```python
from build123d import *

# Parameters (mm, degrees)
SKETCH_1_R          = 4
EXTRUDE_1_DEPTH     = 6.6
SKETCH_2_R          = 4.55
EXTRUDE_2_DEPTH     = 0.2
SKETCH_5_W          = 0.8
SKETCH_5_H          = 0.992889455
EXTRUDE_4_DEPTH     = 0.2
SKETCH_4_R          = 2.4
CUT_EXTRUDE_1_DEPTH = 0.3
FILLET_1_R          = 0.5
SKETCH_3_R          = 0.125
EXTRUDE_3_DEPTH     = 8


with BuildPart() as part:
    # 草图1 → 凸台-拉伸1 (new body)
    with BuildSketch(Plane(origin=(0, 0, 0), x_dir=(1, 0, 0), z_dir=(0, 1, 0))):
        with Locations(Location((0, 0, 0), (0, 0, 270))):
            Circle(SKETCH_1_R)
    extrude(amount=EXTRUDE_1_DEPTH)

    # 草图2 → 凸台-拉伸2 (add)
    with BuildSketch(Plane.XZ):
        with Locations(Location((0, 0, 0), (0, 0, 270))):
            Circle(SKETCH_2_R)
    extrude(amount=EXTRUDE_2_DEPTH)

    # 草图5 → 凸台-拉伸4 (add)
    with BuildSketch(Plane.XZ.offset(0.2)):
        with Locations((0, 4.725827174)):
            Rectangle(SKETCH_5_W, SKETCH_5_H)
    extrude(amount=-EXTRUDE_4_DEPTH)

    # 草图4 → 切除-拉伸1 (cut)
    with BuildSketch(Plane(origin=(0, 6.6, 0), x_dir=(1, 0, 0), z_dir=(0, 1, 0))):
        with Locations(Location((0, 0, 0), (0, 0, 270))):
            Circle(SKETCH_4_R)
    extrude(amount=-CUT_EXTRUDE_1_DEPTH, mode=Mode.SUBTRACT)

    # 圆角1
    fillet_1_edges = [part.edges().sort_by_distance(p)[0] for p in [
        (0, 6.6, -4),
    ]]
    fillet(fillet_1_edges, radius=FILLET_1_R)

    # 草图3 → 凸台-拉伸3 (add)
    with BuildSketch(Plane.XZ.offset(0.2)):
        with Locations(Location((-1.55, 1.55, 0), (0, 0, 270))):
            Circle(SKETCH_3_R)
        with Locations(Location((1.55, 1.55, 0), (0, 0, 90))):
            Circle(SKETCH_3_R)
        with Locations(Location((1.55, -1.55, 0), (0, 0, 270))):
            Circle(SKETCH_3_R)
        with Locations(Location((-1.55, -1.55, 0), (0, 0, 90))):
            Circle(SKETCH_3_R)
    extrude(amount=EXTRUDE_3_DEPTH)


solid = part.part
```
Model file for the job. Use its own axes, mm. Coordinates: 2 decimals unless noted, no trailing zeros. Write each loop counter-clockwise with the first axis right and the second up, starting at its lowest first coordinate (ties: lowest second). Pieces come first, ordered by that corner, then holes. Notation, with made-up numbers: (55, 42.5) - (91, 42.5) arc R19 cw to (91, 66.5) - close; hole circle Ø8 at (-20.5, 83). An arc over 180 degrees is marked (long way). Use a Markdown table: item, result. Add a question column.
Item 1: Drop flat-ended pins along their axis: pin 1 (1.5 mm diameter, centred on x = 2.5, y = 2, fed in from -Z); pin 2 (3 mm diameter, centred on x = -3, z = 4, fed in from -Y); pin 3 (5 mm diameter, centred on x = -1.5, y = -2.5, fed in from +Z). Give the stop position or say it passes through.
Item 2: Band-saw the part on B-B, the plane y = -0.75. Write the cut outline in (x, z) (3 decimals), and give its area (3 significant figures).
Item 3: Two-plate mould, pull along X, no slides. Class faces 1 (the face through (2.04, 0, 3.62)), 2 (the face through (-3.905, 3.007, -0.867)), 3 (the face through (1.62, 6.45, -1.77)): pulls with the +X half, pulls with the -X half, needs draft (parallel to the pull), parting line crosses it, or undercut.
Item 4: Drill centre lines: line 1 along Y through (x, z) = (2.75, 0.75); line 2 along Y through (x, z) = (1.25, 1.5); line 3 along X through (y, z) = (6.4, 0). Where is each one in solid material? Low to high.
Item 5: Band-saw the part on A-A, the plane z = 0. Write the cut outline in (x, y).
Item 6: Band-saw the part on C-C, the plane z = 4.75. Write the cut outline in (x, y).
A:
| question | item | result |
|---|---|---|
| 1 | pin 1 | stops at z = -3.6 |
| 1 | pin 2 | stops at y = -0.2 |
| 1 | pin 3 | stops at z = 4.52 |
| 2 | outline | circle Ø0.25 at (-1.55, -1.55); circle Ø0.25 at (-1.55, 1.55); circle Ø0.25 at (1.55, -1.55); circle Ø0.25 at (1.55, 1.55) |
| 2 | area | 0.196 mm² |
| 3 | face 1 | needs draft |
| 3 | face 2 | parting line crosses it |
| 3 | face 3 | undercut |
| 4 | line 1 | y = -0.2 to 6.6 |
| 4 | line 2 | y = -0.2 to 6.3 |
| 4 | line 3 | x = -3.9 to -2.4, 2.4 to 3.9 |
| 5 | outline | (-4.55, -0.2) - (4.55, -0.2) - (4.55, 0) - (4, 0) - (4, 6.1) arc R0.5 ccw to (3.5, 6.6) - (2.4, 6.6) - (2.4, 6.3) - (-2.4, 6.3) - (-2.4, 6.6) - (-3.5, 6.6) arc R0.5 ccw to (-4, 6.1) - (-4, 0) - (-4.55, 0) - close |
| 6 | outline | (-0.4, -0.2) - (0.4, -0.2) - (0.4, 0) - (-0.4, 0) - close |
